The figure shows three views and two pictorial views of one solid part (mm, origin at its lowest corner). Answer the questions. A direction names the side the tool comes from. Give positions to 0.01 mm unless a question says otherwise; leave off trailing zeros. Write each loop counter-clockwise with the first axis right and the second up, starting at its lowest first coordinate (ties: lowest second). Pieces come first, ordered by that corner, then holes. Notation, with made-up numbers: (-39, -10) -> (9, -10) arc R13 ccw to (9, 15) -> close; hole circle Ø9 at (-4, 55). An arc over 180 degrees is marked (long way). Use a Markdown table: item, result.
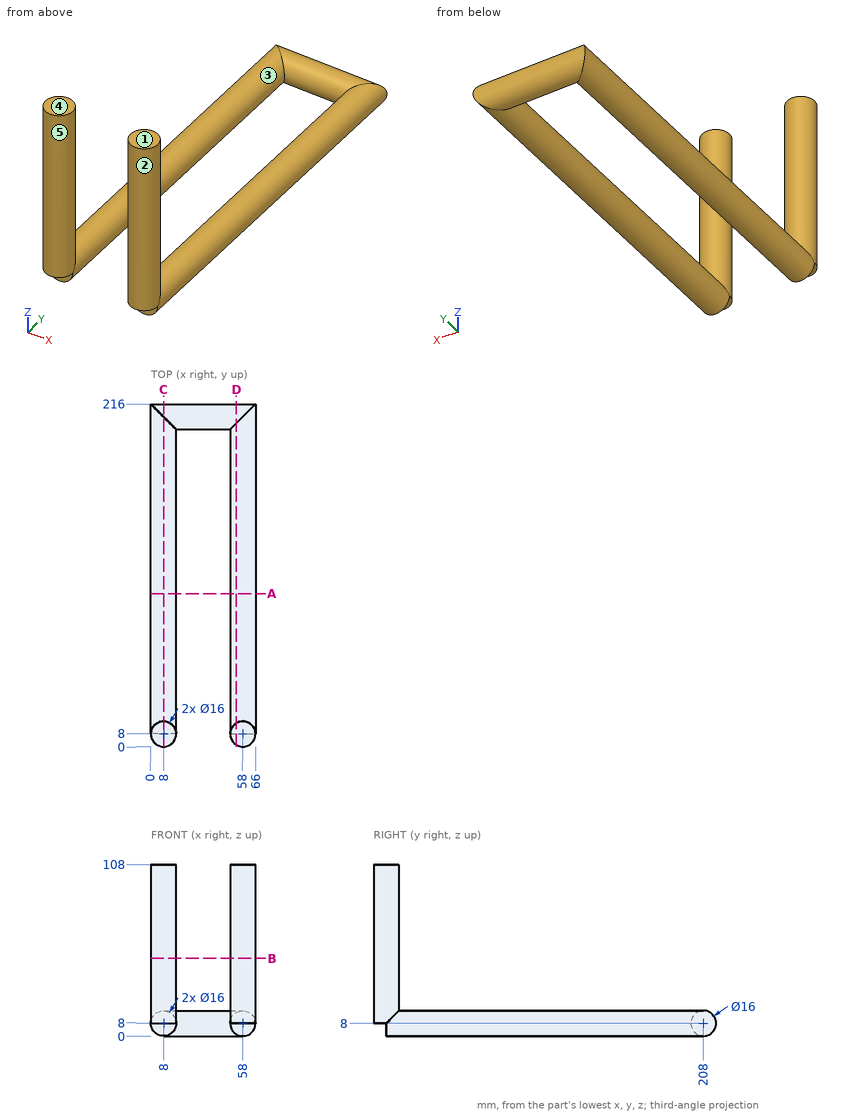
Item 1: A cutting plane is placed at C-C (x = 8). Give the vertices of the cut face in (y, z).
Return value:
| item | result |
|---|---|
| outline | (0, 8) -> (8, 8) -> (8, 0) -> (208, 0) arc R8 ccw to (208, 16) -> (16, 16) -> (16, 108) -> (0, 108) -> close |
Item 2: Straight lines are drawn through the part: line 1 along X through (y, z) = (182, 14); line 2 along Y through (x, z) = (8, 38.5); line 3 along X through (y, z) = (160, 11). For each, find the intervals that lie inside material, in ascending order. Write a range as [from, to].
Return value:
| item | result |
|---|---|
| line 1 | [2.71, 13.29], [52.71, 63.29] |
| line 2 | [0, 16] |
| line 3 | [0.58, 15.42], [50.58, 65.42] |
Item 3: A tool of negligible diameter and unlimited length cuts with its end or side. For the marked faces 3, 4 and 5, from which of +Z, -Z, +X, -X, +Y, -Y can it reach the whole face along a straight path? Write none if from no direction.
Return value:
| item | result |
|---|---|
| face 3 | none |
| face 4 | +Z, +X, -X, +Y, -Y |
| face 5 | +Z |
Item 4: A cutting plane is placed at D-D (x = 54). Give the vertices of the cut face in (y, z).
Return value:
| item | result |
|---|---|
| outline | (1.07, 8) -> (8, 8) -> (8, 1.07) -> (204, 1.07) arc R8 ccw (long way) to (204, 14.93) -> (14.93, 14.93) -> (14.93, 108) -> (1.07, 108) -> close |
Item 5: For a pull along X with two mould halves and no side action, classify the marked faces 1 and 2 as +X half, -X half, draft (parallel to the pull), parting line (faces both ways), or undercut.
Return value:
| item | result |
|---|---|
| face 1 | draft |
| face 2 | undercut |
Item 6: A cutting plane is placed at A-A (y = 96.5). Give the vertices of the cut face in (x, z).
Return value:
| item | result |
|---|---|
| outline | circle Ø16 at (8, 8); circle Ø16 at (58, 8) |
Item 7: Each of these flat-tipped pins is pushed along its axis until it touches: P1, Ø6.5, axis at x = 11, z = 4, coming from the -Y side; P2, Ø12, axis at x = 49, y = 68.5, coming from the +Z side; P3, Ø6, axis at x = 16.5, y = 193, coming from the -Z side. Where does it stop, or does it pass through?
Return value:
| item | result |
|---|---|
| P1 | y = 8 |
| P2 | z = 15.42 |
| P3 | z = 2.19 |
